```python
from build123d import *

# Parameters (mm, degrees)
SKETCH1_R           = 3.175
BOSS_EXTRUDE1_DEPTH = 3.175
FILLET1_R           = 2.54
BOSS_EXTRUDE2_DEPTH = 6.35


with BuildPart() as part:
    # Sketch1 → Boss-Extrude1 (new, symmetric)
    with BuildSketch(Plane.XY):
        with BuildLine():
            Line((8.255, 0), (8.255, -144.145))
            ThreePointArc((8.255, -144.145), (5.837166479, -149.982166479), (0, -152.4))
            Line((0, -152.4), (-28.575, -152.4))
            Line((-28.575, -152.4), (-28.575, -127))
            Line((-28.575, -127), (-15.875, -127))
            Line((-15.875, -127), (-15.875, -130.81))
            ThreePointArc((-15.875, -130.81), (-15.131051224, -132.606051224), (-13.335, -133.35))
            Line((-13.335, -133.35), (-5.715, -133.35))
            ThreePointArc((-5.715, -133.35), (-3.918948776, -132.606051224), (-3.175, -130.81))
            Line((-3.175, -130.81), (-3.175, -71.12))
            ThreePointArc((-3.175, -71.12), (-8.255, -63.5), (-3.175, -55.88))
            Line((-3.175, -55.88), (-3.175, -7.62))
            ThreePointArc((-3.175, -7.62), (-4.57905012, 6.86857518), (8.255, 0))
        make_face()
        Circle(SKETCH1_R, mode=Mode.SUBTRACT)
        with Locations((0, -63.5)):
            Circle(SKETCH1_R, mode=Mode.SUBTRACT)
    extrude(amount=BOSS_EXTRUDE1_DEPTH, both=True)

    # Fillet1
    fillet1_edges = [part.edges().sort_by_distance(p)[0] for p in [
        (-3.175, -7.62, 0),
    ]]
    fillet(fillet1_edges, radius=FILLET1_R)

    # Sketch2 → Boss-Extrude2 (add)
    with BuildSketch(Plane.XY.offset(3.175)):
        with BuildLine():
            Line((14.605, -70.822423777), (14.605, -77.172423777))
            ThreePointArc((14.605, -77.172423777), (17.78, -80.347423777), (20.955, -77.172423777))
            Line((20.955, -77.172423777), (20.955, -70.822423777))
            ThreePointArc((20.955, -70.822423777), (19.207129933, -65.323162463), (14.605, -61.842167656))
            ThreePointArc((14.605, -61.842167656), (10.002870067, -58.361172848), (8.255, -52.861911534))
            Line((8.255, -52.861911534), (8.255, -70.822423777))
            ThreePointArc((8.255, -70.822423777), (11.43, -67.647423777), (14.605, -70.822423777))
        make_face()
    extrude(amount=-BOSS_EXTRUDE2_DEPTH)


solid = part.part
```
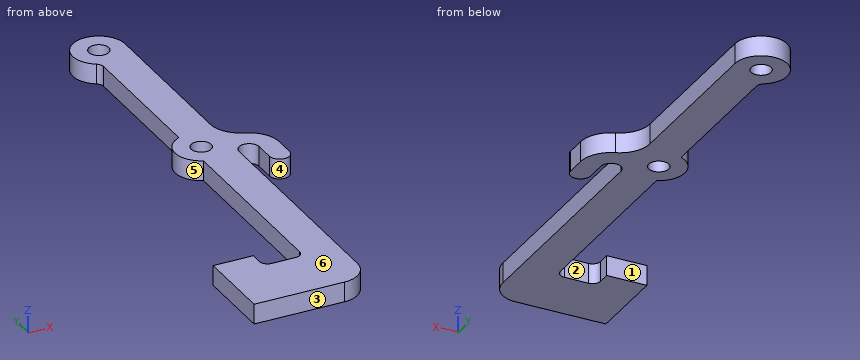
CAD build for the part. Positions are in the model's coordinates, mm. Face numbers are marked on the shaded views. A direction names the side the tool comes from. Round coordinates to 2 decimals unless told otherwise and drop trailing zeros. Order: outer loops, then holes, each group sorted by start corner. A loop starts at its lowest first (then second) coordinate and runs counter-clockwise, first axis right, second up.
Item 1: Probe line 1 along Y through (x, z) = (0, -0.25) (3 decimals); line 2 along Y through (x, z) = (-7.5, -1.5); line 3 along X through (y, z) = (-94, 1.5) (3 decimals). List the from-to ranges inside material, lowest first.
Item 2: Pin check, flat tips, straight feed: pin 1 (10 mm diameter, centred on x = -13, y = -44, fed in from -Z); pin 2 (3 mm diameter, centred on y = -13, z = 2.5, fed in from -X) (3 decimals); pin 3 (2 mm diameter, centred on x = -15, z = -1, fed in from +Y); pin 4 (1.5 mm diameter, centred on y = -135, z = 2.5, fed in from +X) (3 decimals). Stop position of each tip, or through.
Item 3: Saw through at A-A on z = -1.75. Write the cut outline in (x, y) (3 decimals).
Item 4: Saw through at B-B on y = -63.5. Write the cut outline in (x, z) (3 decimals), then the cut area to 3 significant figures.
Item 5: Saw through at C-C on x = 11.43. Write the cut outline in (y, z) (3 decimals), then the cut area to 3 significant figures.
Item 6: Tool access for the marked faces 1, 2 and 3: list every direction of +Z, -Z, +X, -X, +Y, -Y with a clear straight run to the whole face (end or side of a thin tool).
Item 7: Saw through at D-D on y = -138. Write the cut outline in (x, z) (3 decimals), then the cut area to 3 significant figures.
Item 8: Mould opens along Y. For the marked faces 4, 5 and 6 say: pulls with the +Y half, pulls with the -Y half, needs draft (parallel to the pull), parting line crosses it, or undercut.
Reported:
1. line 1: y = -152.4 to -66.675, -60.325 to -3.175, 3.175 to 8.255
1. line 2: y = -152.4 to -133.35, -66.95 to -60.05, -3.45 to 3.45
1. line 3: x = -3.175 to 8.255
2. pin 1: passes through
2. pin 2: stops at x = -3.175
2. pin 3: stops at y = -127
2. pin 4: stops at x = 8.255
3. outline: (-28.575, -152.4) - (0, -152.4) arc R8.255 ccw to (8.255, -144.145) - (8.255, -70.822) arc R3.175 cw to (14.605, -70.822) - (14.605, -77.172) arc R3.175 ccw to (20.955, -77.172) - (20.955, -70.822) arc R9.525 ccw to (14.605, -61.842) arc R9.525 cw to (8.255, -52.862) - (8.255, 0) arc R8.255 ccw (long way) to (-4.37, -7.003) arc R2.54 cw to (-3.175, -9.158) - (-3.175, -55.88) arc R8.255 ccw to (-3.175, -71.12) - (-3.175, -130.81) arc R2.54 cw to (-5.715, -133.35) - (-13.335, -133.35) arc R2.54 cw to (-15.875, -130.81) - (-15.875, -127) - (-28.575, -127) - close; hole circle Ø6.35 at (0, -63.5); hole circle Ø6.35 at (0, 0)
4. outline: (-8.255, -3.175) - (-3.175, -3.175) - (-3.175, 3.175) - (-8.255, 3.175) - close; (3.175, -3.175) - (17.522, -3.175) - (17.522, 3.175) - (3.175, 3.175) - close
4. area: 123 mm2
5. outline: (-67.647, -3.175) - (-59.961, -3.175) - (-59.961, 3.175) - (-67.647, 3.175) - close
5. area: 48.8 mm2
6. face 1: +Z, -Z, -X, +Y
6. face 2: +Z, -Z
6. face 3: +Z, -Z, +X, -X, -Y
7. outline: (-28.575, -3.175) - (8.255, -3.175) - (8.255, 3.175) - (-28.575, 3.175) - close
7. area: 234 mm2
8. face 4: pulls with the -Y half
8. face 5: undercut
8. face 6: needs draft
